```python
from build123d import *

# Parameters (mm, degrees)
F2_R          = 5
F6_DEPTH      = 19.0010001
F6_DEPTH_BACK = 19.0010001
F13_SIZE      = 1


with BuildPart() as f1:
    # F0 (on Front) → F1 (revolve)
    with BuildSketch(Plane.XZ):
        Polygon((0, 0), (0, 19), (-70, 15), (-70, 0), align=None)
    revolve(axis=Axis((-35, 0, 0), (1, 0, 0)))

    # F2
    f2_edges = [f1.edges().sort_by_distance(p)[0] for p in [
        (-70, 0, -15),
    ]]
    fillet(f2_edges, radius=F2_R)

    # F3 (on Top) → F4 (revolve, cut)
    with BuildSketch(Plane.XY):
        with BuildLine():
            Line((-42.5, 6.5), (-70, 6.5))
            Line((-70, 6.5), (-70, -6.5))
            Line((-70, -6.5), (-42.5, -6.5))
            ThreePointArc((-42.5, -6.5), (-36, 0), (-42.5, 6.5))
        make_face()
    revolve(axis=Axis((-70, 10.4297241849, 0), (0, -1, 0)), mode=Mode.SUBTRACT)

    # F5 (on Top) → F6 (cut, two sides)
    with BuildSketch(Plane.XY) as f6_sk:
        Polygon((-23.5, 0), (-70, 0), (-70, -19), (0, -19), (0, 0), (-20.5, 0), (-20.5, -4), (-23.5, -4), align=None)
    extrude(amount=-F6_DEPTH, mode=Mode.SUBTRACT)
    extrude(f6_sk.sketch, amount=F6_DEPTH_BACK, mode=Mode.SUBTRACT)

    # F7 (on Top) → F8 (revolve, cut)
    with BuildSketch(Plane.XY):
        with BuildLine():
            Line((-13.7, 0), (0, 0))
            Line((0, 0), (0, 9.1))
            Line((0, 9.1), (-6.8, 9.1))
            Line((-6.8, 9.1), (-6.8, 12.1))
            ThreePointArc((-6.8, 12.1), (-6.9464466094, 12.4535533906), (-7.3, 12.6))
            Line((-7.3, 12.6), (-13.2, 12.6))
            ThreePointArc((-13.2, 12.6), (-13.5535533906, 12.4535533906), (-13.7, 12.1))
            Line((-13.7, 12.1), (-13.7, 0))
        make_face()
    revolve(axis=Axis((-6.85, 0, 0), (1, 0, 0)), mode=Mode.SUBTRACT)

    # F9 (on Top) → F10 (revolve, cut)
    with BuildSketch(Plane.XY):
        Polygon((-22, 19.2228130501), (-28.8849250614, 19.2228130501), (-27.1, 9.1), (-27.1, -4), (-22, -4), align=None)
    revolve(axis=Axis((-22, 7.6114065251, 0), (0, -1, 0)), mode=Mode.SUBTRACT)

    # F11 (on Top) → F12 (revolve, cut)
    with BuildSketch(Plane.XY):
        Polygon((-56, 6.5), (-56, 21.9801377317), (-63.7295659472, 21.9801377317), (-61, 6.5), align=None)
    revolve(axis=Axis((-56, 14.2400688658, 0), (0, 1, 0)), mode=Mode.SUBTRACT)

    # F13
    f13_edges = [f1.edges().sort_by_distance(p)[0] for p in [
        (-6.8, 9.1, 0),
        (0, 9.1, 0),
    ]]
    chamfer(f13_edges, length=F13_SIZE)


solid = f1.part
```
Design review of the part built by this model. Coordinates are the model's own, in mm. A direction names the side the tool comes from. Round coordinates to 2 decimals unless told otherwise and drop trailing zeros. Order: outer loops, then holes, each group sorted by start corner. A loop starts at its lowest first (then second) coordinate and runs counter-clockwise, first axis right, second up. Notation, with made-up numbers: (57.5, 62) - (98.5, 62) arc R24 ccw to (98.5, 75) - close; hole circle Ø7 at (-4, -35). An arc over 180 degrees is marked (long way). One line per question, with ' | ' between items.
Item 1: Draft analysis for pull direction X (two halves, no side actions). For faces 1 (the face through (-51.515, 10.198, -3.439)), 2 (the face through (-16.905, 3.914, -0.224)), 3 (the face through (-15, 0, 0)), 4 (the face through (-70, 8, 0)), state which applies: +X half, -X half, draft (parallel to the pull), parting line (faces both ways), or undercut.
Checks:
face 1: undercut | face 2: undercut | face 3: draft | face 4: -X half
Item 2: Take a section at B-B, the plane z = 0. Write out the cut boundary in (x, y), then the cut area to 3 significant figures.
Checks:
outline: (-70, 6.5) - (-61, 6.5) - (-62.57, 15.42) - (-65.29, 15.27) arc R5 ccw to (-70, 10.28) - close; (-51, 6.5) - (-42.5, 6.5) arc R6.5 cw to (-36, 0) - (-27.1, 0) - (-27.1, 9.1) - (-28.56, 17.37) - (-49.29, 16.18) - close; (-16.9, 0) - (-13.7, 0) - (-13.7, 12.1) arc R0.5 cw to (-13.2, 12.6) - (-7.3, 12.6) arc R0.5 cw to (-6.8, 12.1) - (-6.8, 10.1) - (-5.8, 9.1) - (-1, 9.1) - (0, 10.1) - (0, 19) - (-15.31, 18.13) - (-16.9, 9.1) - close | area: 521 mm²
Item 3: For P1, Ø1, axis at x = -8, y = 2, coming from the +Z side; P2, Ø4, axis at y = 13, z = -5.5, coming from the -X side; P3, Ø1, axis at y = 7, z = 14, coming from the +X side; P4, Ø10, axis at x = -42.5, z = -12, coming from the +Y side, all flat-tipped, find the tip position at first contact; note any pin that passes through.
Checks:
P1: z = 18.49 | P2: x = -69.65 | P3: x = 0 | P4: y = 15.04
Item 4: Take a section at C-C, the plane y = 8.25. Give the number of separate pieces and of enclosed holes in the cut face, then the cut area to 3 significant figures.
Checks:
separate pieces: 1 | enclosed holes: 2 | area: 1,710 mm²
Item 5: Take a section at D-D, the plane x = -14.5. Write out the cut boundary in (y, z).
Checks:
outline: (0, -18.17) arc R18.17 ccw to (0, 18.17) - close
Item 6: Machinability: for faces 5 (the face through (-32, 0, 0)), 6 (the face through (-3.434, 9.098, -0.2)), 7 (the face through (-20.5, -2, 11)), 8 (the face through (-13.7, 5, 0)), which of the approach directions +Z, -Z, +X, -X, +Y, -Y give a long, thin tool a straight path to every point of the face, cutting with its end or side? Answer none if there is none.
Checks:
face 5: +Z, -Z, -X, -Y | face 6: +X, -Y | face 7: +Z, -Z, +X, -Y | face 8: -Y
Item 7: Wall thickness on line 1 (X direction, y = 0.5, z = 0); line 2 (X direction, y = 3.25, z = -9); line 3 (Z direction, x = -22, y = 2): over which ranges is each line inside the solid? List them lowest first. Write a range as [from, to].
Checks:
line 1: [-36.02, -27.1], [-16.9, -13.7] | line 2: [-38.12, -13.7], [-6.27, -0.53] | line 3: [-17.63, -5.1], [5.1, 17.63]
Item 8: Take a section at A-A, the plane x = -22. Write out the cut boundary in (y, z), then the cut area to 3 significant figures.
Checks:
outline: (-4, -17.29) arc R17.74 ccw to (16.54, -6.41) - (9.1, -5.1) - (-4, -5.1) - close; (-4, 5.1) - (9.1, 5.1) - (16.54, 6.41) arc R17.74 ccw to (-4, 17.29) - close | area: 406 mm²
